Here's how the part is built. I have some questions about the finished solid (model axes, mm). Face numbers are marked on the shaded views. A direction names the side the tool comes from. Coordinates: 2 decimals unless noted, no trailing zeros. Write each loop counter-clockwise with the first axis right and the second up, starting at its lowest first coordinate (ties: lowest second). Pieces come first, ordered by that corner, then holes. Notation, with made-up numbers: (27, 16.5) -> (64, 16.5) arc R7 cw to (64, 23.5) -> close; hole circle Ø4 at (67.5, 79). An arc over 180 degrees is marked (long way). Use a Markdown table: item, result. Add a question column.
```python
from build123d import *

# Parameters (mm, degrees)
SKETCH1_R           = 12.5
BOSS_EXTRUDE1_DEPTH = 3.5


with BuildPart() as part:
    # Sketch1 → Boss-Extrude1 (new body, symmetric)
    with BuildSketch(Plane.XY):
        Circle(SKETCH1_R)
        with BuildLine():
            Line((1, -1), (-1, -1))
            ThreePointArc((-1, -1), (-2, 0), (-1, 1))
            Line((-1, 1), (1, 1))
            ThreePointArc((1, 1), (2, 0), (1, -1))
        make_face(mode=Mode.SUBTRACT)
    extrude(amount=BOSS_EXTRUDE1_DEPTH, both=True)


solid = part.part
```
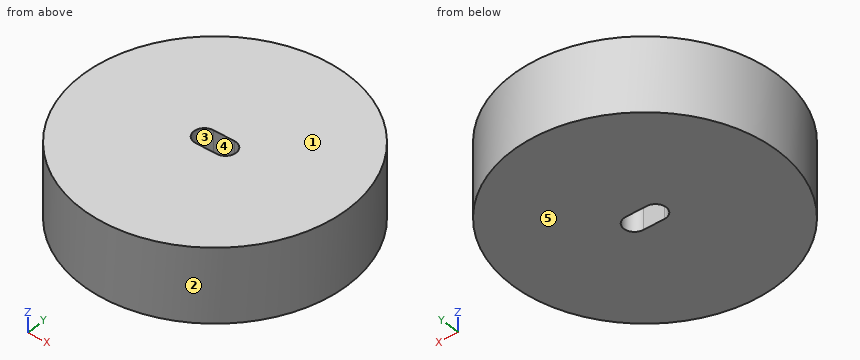
Q1. Suppose I cut it at A-A, the plane y = 0. Write out the boundary of the cut face in (x, z), and give its area (3 significant figures).
Q2. Suppose I cut it at C-C, the plane x = 7.5. Write out the boundary of the cut face in (y, z), and give its area (3 significant figures).
Q3. Will these pins go through, and if not, where does the flat tip stop? pin 1 (4 mm diameter, centred on y = -7.5, z = 1.5, fed in from +X) (3 decimals); pin 2 (2 mm diameter, centred on x = 3.5, z = -1, fed in from -Y); pin 3 (3 mm diameter, centred on x = -3.5, z = 1, fed in from +Y).
Q4. Please list where these lines run through material, in increasing order: line 1 (Y direction, x = -1.5, z = -0.5); line 2 (X direction, y = -11, z = 0.75); line 3 (Y direction, x = -5, z = 1.25).
Q5. Thinking about a two-plate mould opening in Y: for the marked faces 1, 2 and 3, which applies, released by +Y, released by -Y, zero draft, split by the parting line, or undercut?
Q6. Suppose I cut it at B-B, the plane x = 0. Write out the boundary of the cut face in (y, z).
Q7. Which directions (+Z, -Z, +X, -X, +Y, -Y) give clear straight access to the entire face, cutting with the end or side of a thin tool? Please do the marked faces 4 and 5.
Q8. Suppose I cut it at D-D, the plane y = -3. Write out the boundary of the cut face in (x, z).
Answer key:
| question | item | result |
|---|---|---|
| 1 | outline | (-12.5, -3.5) -> (-2, -3.5) -> (-2, 3.5) -> (-12.5, 3.5) -> close; (2, -3.5) -> (12.5, -3.5) -> (12.5, 3.5) -> (2, 3.5) -> close |
| 1 | area | 147 mm^2 |
| 2 | outline | (-10, -3.5) -> (10, -3.5) -> (10, 3.5) -> (-10, 3.5) -> close |
| 2 | area | 140 mm^2 |
| 3 | pin 1 | stops at x = 11.225 |
| 3 | pin 2 | stops at y = -12.25 |
| 3 | pin 3 | stops at y = 12.34 |
| 4 | line 1 | y = -12.41 to -0.87, 0.87 to 12.41 |
| 4 | line 2 | x = -5.94 to 5.94 |
| 4 | line 3 | y = -11.46 to 11.46 |
| 5 | face 1 | zero draft |
| 5 | face 2 | split by the parting line |
| 5 | face 3 | undercut |
| 6 | outline | (-12.5, -3.5) -> (-1, -3.5) -> (-1, 3.5) -> (-12.5, 3.5) -> close; (1, -3.5) -> (12.5, -3.5) -> (12.5, 3.5) -> (1, 3.5) -> close |
| 7 | face 4 | +Z, -Z |
| 7 | face 5 | -Z, +X, -X, +Y, -Y |
| 8 | outline | (-12.13, -3.5) -> (12.13, -3.5) -> (12.13, 3.5) -> (-12.13, 3.5) -> close |
